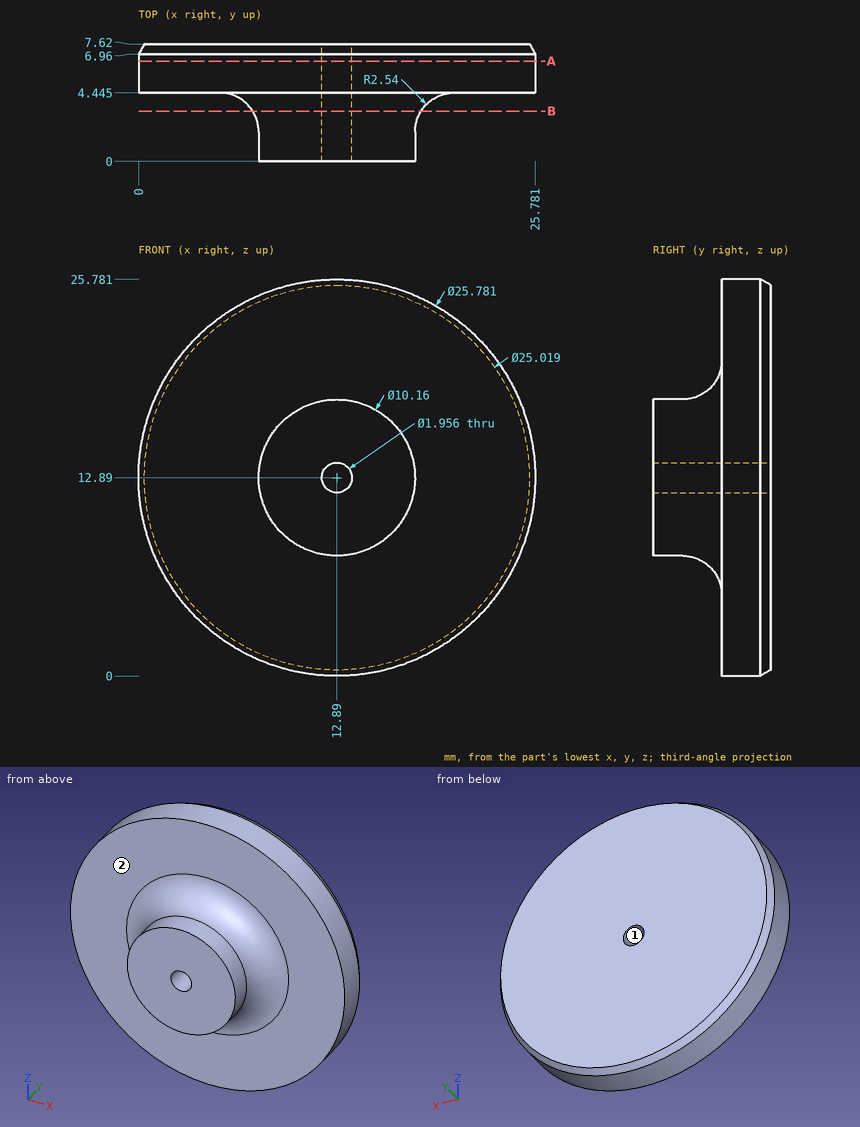
Study the drawing (mm; zero at the part's minimum x, y, z) and answer. A direction names the side the tool comes from. Coordinates: 2 decimals unless noted, no trailing zeros. Loops run counter-clockwise (first coordinate to the right, second up) from the corner with the lowest first, then second, coordinate; pieces in that order, holes last. Notation, with made-up numbers: (-21.5, 36.25) -> (-17.5, 36.25) arc R28 cw to (-17.5, 56.25) -> close; hole circle Ø6 at (10, 49). An arc over 180 degrees is marked (long way). Answer as CSV lines item,"result".
1) For the marked faces 1 and 2, determine the directions among +Z, -Z, +X, -X, +Y, -Y from which every point of the face is accessible in a straight line to the end or side of a thin tool.
A:
face 1,"+Y, -Y"
face 2,"-Y"
2) Straight lines are drawn through the part: probe 1 along Y at (x, z) = (3.5, 20.75) (1 decimal); probe 2 along X at (y, z) = (7, 13) (1 decimal); probe 3 along X at (y, z) = (4, 11.5) (1 decimal). For each, find the intervals that lie inside material, in ascending order.
A:
probe 1,"y = 4.4 to 7.6"
probe 2,"x = 0 to 11.9, 13.9 to 25.8"
probe 3,"x = 6.9 to 18.9"
3) The part is cut by section A-A (y = 6.5). Give the vertices of the cut face in (x, z) (1 decimal), and give its area (3 significant figures).
A:
outline,"circle Ø25.8 at (12.9, 12.9); hole circle Ø2 at (12.9, 12.9)"
area,"519 mm²"
4) Flat-ended cylindrical pins translate along their axes: pin 1 (3 mm diameter, centred on y = 3.5, z = 6.5, fed in from -X); pin 2 (8 mm diameter, centred on x = 23, z = 23, fed in from +Y); pin 3 (1 mm diameter, centred on x = 12, y = 4, fed in from -Z); pin 4 (1.5 mm diameter, centred on y = 4.5, z = 8.5, fed in from -X) (1 decimal). Find the tip coordinate at first contact, or state that the pin passes through.
A:
pin 1,"stops at x = 1.11"
pin 2,"stops at y = 7.62"
pin 3,"stops at z = 0.02"
pin 4,"stops at x = 0.5"
5) The part is cut by section B-B (y = 3.25). Give the vertices of the cut face in (x, z) (1 decimal).
A:
outline,"circle Ø10.9 at (12.9, 12.9); hole circle Ø2 at (12.9, 12.9)"
